Part model, mm, in its own coordinate system. Face numbers are marked on the shaded views. A direction names the side the tool comes from. Coordinates: 2 decimals unless noted, no trailing zeros. Write each loop counter-clockwise with the first axis right and the second up, starting at its lowest first coordinate (ties: lowest second). Pieces come first, ordered by that corner, then holes. Notation, with made-up numbers: (8.25, 35.25) - (25.25, 35.25) arc R29 ccw to (25.25, 62.25) - close; hole circle Ø11 at (-15, 45.5). An arc over 180 degrees is marked (long way). Use a Markdown table: item, result.
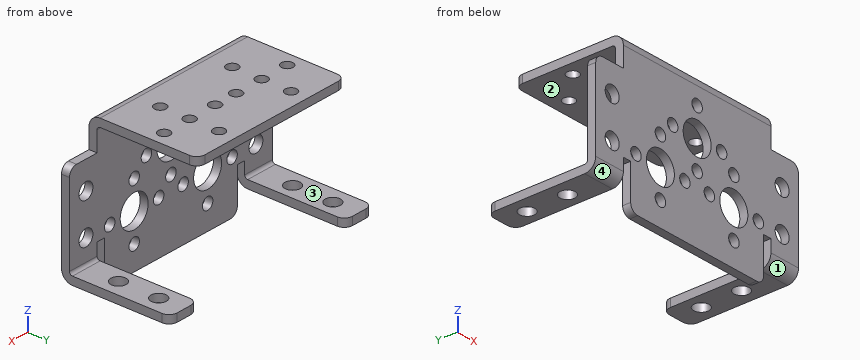
```python
from build123d import *

# Parameters (mm, degrees)
SM_BASE_FLANGE_1_DEPTH             = 2
SM_EDGE_FLANGE_1_STRIP_W           = 9.4732
SM_EDGE_FLANGE_1_STRIP_H           = 2
SM_EDGE_FLANGE_1_STRIP_CUT_DEPTH   = 42.2
SM_EDGE_FLANGE_1_DEPTH             = 42.2
SM_START                           = 2
SM_EDGE_FLANGE_1_FLAT_DEPTH        = 2
SM_EDGE_FLANGE_2_STRIP_W           = 9.4732
SM_EDGE_FLANGE_2_STRIP_H           = 2
SM_EDGE_FLANGE_2_STRIP_CUT_DEPTH   = 7.9
SM_EDGE_FLANGE_2_STRIP_2_W         = 9.4732
SM_EDGE_FLANGE_2_STRIP_2_H         = 2
SM_EDGE_FLANGE_2_STRIP_CUT_2_DEPTH = 7.9
SM_EDGE_FLANGE_2_DEPTH             = 7.9
SM_EDGE_FLANGE_2_PROFILE_R         = 1.9
SM_EDGE_FLANGE_2_FLAT_DEPTH        = 2
SM_EDGE_FLANGE_2_BEND_DEPTH        = 7.9
SM_EDGE_FLANGE_2_PROFILE_2_R       = 1.9
SM_EDGE_FLANGE_2_FLAT_2_DEPTH      = 2
HOLE_WIZARD_8_0_8_1_D              = 8
HOLE_WIZARD_3_0_3_1_D              = 3
HOLE_WIZARD_4_0_4_1_D              = 4
HOLE_WIZARD_2_9_2_9_2_D            = 2.9


# Sheet-metal steps are written as plain solids
with BuildPart() as part:
    # Sketch 2 → 基体-法兰1 (new body)
    with BuildSketch(Plane(origin=(0, 0, 0), x_dir=(1, 0, 0), z_dir=(0, 1, 0))):
        with BuildLine():
            Line((-17, 23.49), (17, 23.49))
            ThreePointArc((17, 23.49), (18.414213562, 22.904213562), (19, 21.49))
            Line((19, 21.49), (19, 12.7))
            Line((19, 12.7), (21.1, 12.7))
            Line((21.1, 12.7), (21.1, 16.5))
            Line((21.1, 16.5), (29, 16.5))
            Line((29, 16.5), (29, -4.3))
            ThreePointArc((29, -4.3), (28.414213562, -5.714213562), (27, -6.3))
            Line((27, -6.3), (21.1, -6.3))
            Line((21.1, -6.3), (21.1, -12))
            Line((21.1, -12), (-21.1, -12))
            Line((-21.1, -12), (-21.1, -6.3))
            Line((-21.1, -6.3), (-27, -6.3))
            ThreePointArc((-27, -6.3), (-28.414213562, -5.714213562), (-29, -4.3))
            Line((-29, -4.3), (-29, 16.5))
            Line((-29, 16.5), (-21.1, 16.5))
            Line((-21.1, 16.5), (-21.1, 12.7))
            Line((-21.1, 12.7), (-19, 12.7))
            Line((-19, 12.7), (-19, 21.49))
            ThreePointArc((-19, 21.49), (-18.414213562, 22.904213562), (-17, 23.49))
        make_face()
    extrude(amount=-SM_BASE_FLANGE_1_DEPTH)

    # 边线-法兰1 strip (across the edge) → 边线-法兰1 strip cut (cut)
    with BuildSketch(Plane(origin=(-21.1, 0, 12), x_dir=(0, 0, -1), z_dir=(1, 0, 0))):
        with Locations((-4, -1)):
            Rectangle(SM_EDGE_FLANGE_1_STRIP_W, SM_EDGE_FLANGE_1_STRIP_H)
    extrude(amount=SM_EDGE_FLANGE_1_STRIP_CUT_DEPTH, mode=Mode.SUBTRACT)

    # 边线-法兰1 bend section (across the edge) → 边线-法兰1 (add)
    with BuildSketch(Plane(origin=(-21.1, 0, 12), x_dir=(0, 0, -1), z_dir=(1, 0, 0))):
        with BuildLine():
            Line((-2, 0.7366), (0, 0.7366))
            ThreePointArc((0, 0.7366), (0.215745145, 0.215745145), (0.7366, 0))
            Line((0.7366, 0), (0.7366, -2))
            ThreePointArc((0.7366, -2), (-1.198468417, -1.198468417), (-2, 0.7366))
        make_face()
    extrude(amount=SM_EDGE_FLANGE_1_DEPTH)

    # 边线-法兰1 profile (on flange) → 边线-法兰1 flat (add)
    with BuildSketch(Plane.XY.offset(12).offset(SM_START)):
        with BuildLine():
            Line((-21.1, 0.7366), (21.1, 0.7366))
            Line((21.1, 0.7366), (21.1, 23))
            ThreePointArc((21.1, 23), (20.514213562, 24.414213562), (19.1, 25))
            Line((19.1, 25), (-19.1, 25))
            ThreePointArc((-19.1, 25), (-20.514213562, 24.414213562), (-21.1, 23))
            Line((-21.1, 23), (-21.1, 0.7366))
        make_face()
    extrude(amount=-SM_EDGE_FLANGE_1_FLAT_DEPTH)

    # 边线-法兰2 strip (across the edge) → 边线-法兰2 strip cut (cut)
    with BuildSketch(Plane(origin=(-21.1, 0, -16.5), x_dir=(0, 0, 1), z_dir=(-1, 0, 0))):
        with Locations((-4, -1)):
            Rectangle(SM_EDGE_FLANGE_2_STRIP_W, SM_EDGE_FLANGE_2_STRIP_H)
    extrude(amount=SM_EDGE_FLANGE_2_STRIP_CUT_DEPTH, mode=Mode.SUBTRACT)

    # 边线-法兰2 strip 2 (across the edge) → 边线-法兰2 strip cut 2 (cut)
    with BuildSketch(Plane(origin=(29, 0, -16.5), x_dir=(0, 0, 1), z_dir=(-1, 0, 0))):
        with Locations((-4, -1)):
            Rectangle(SM_EDGE_FLANGE_2_STRIP_2_W, SM_EDGE_FLANGE_2_STRIP_2_H)
    extrude(amount=SM_EDGE_FLANGE_2_STRIP_CUT_2_DEPTH, mode=Mode.SUBTRACT)

    # 边线-法兰2 bend section (across the edge) → 边线-法兰2 (add)
    with BuildSketch(Plane(origin=(-21.1, 0, -16.5), x_dir=(0, 0, 1), z_dir=(-1, 0, 0))):
        with BuildLine():
            Line((-2, 0.7366), (0, 0.7366))
            ThreePointArc((0, 0.7366), (0.215745145, 0.215745145), (0.7366, 0))
            Line((0.7366, 0), (0.7366, -2))
            ThreePointArc((0.7366, -2), (-1.198468417, -1.198468417), (-2, 0.7366))
        make_face()
    extrude(amount=SM_EDGE_FLANGE_2_DEPTH)

    # 边线-法兰2 profile (on flange) → 边线-法兰2 flat (add)
    with BuildSketch(Plane(origin=(0, 0, -16.5), x_dir=(-1, 0, 0), z_dir=(0, 0, -1)).offset(SM_START)):
        with BuildLine():
            ThreePointArc((23.1, 25), (21.685786438, 24.414213562), (21.1, 23))
            Line((21.1, 23), (21.1, 0.7366))
            Line((21.1, 0.7366), (29, 0.7366))
            Line((29, 0.7366), (29, 23))
            ThreePointArc((29, 23), (28.414213562, 24.414213562), (27, 25))
            Line((27, 25), (23.1, 25))
        make_face()
        with Locations((24.9, 8.6)):
            Circle(SM_EDGE_FLANGE_2_PROFILE_R, mode=Mode.SUBTRACT)
        with Locations((24.9, 18.6)):
            Circle(SM_EDGE_FLANGE_2_PROFILE_R, mode=Mode.SUBTRACT)
    extrude(amount=-SM_EDGE_FLANGE_2_FLAT_DEPTH)

    # 边线-法兰2 bend section 2 (across the edge) → 边线-法兰2 bend (add)
    with BuildSketch(Plane(origin=(29, 0, -16.5), x_dir=(0, 0, 1), z_dir=(-1, 0, 0))):
        with BuildLine():
            Line((-2, 0.7366), (0, 0.7366))
            ThreePointArc((0, 0.7366), (0.215745145, 0.215745145), (0.7366, 0))
            Line((0.7366, 0), (0.7366, -2))
            ThreePointArc((0.7366, -2), (-1.198468417, -1.198468417), (-2, 0.7366))
        make_face()
    extrude(amount=SM_EDGE_FLANGE_2_BEND_DEPTH)

    # 边线-法兰2 profile 2 (on flange) → 边线-法兰2 flat 2 (add)
    with BuildSketch(Plane(origin=(0, 0, -16.5), x_dir=(-1, 0, 0), z_dir=(0, 0, -1)).offset(SM_START)):
        with BuildLine():
            Line((-29, 23), (-29, 0.7366))
            Line((-29, 0.7366), (-21.1, 0.7366))
            Line((-21.1, 0.7366), (-21.1, 23))
            ThreePointArc((-21.1, 23), (-21.685786438, 24.414213562), (-23.1, 25))
            Line((-23.1, 25), (-27, 25))
            ThreePointArc((-27, 25), (-28.414213562, 24.414213562), (-29, 23))
        make_face()
        with Locations((-24.9, 8.6)):
            Circle(SM_EDGE_FLANGE_2_PROFILE_2_R, mode=Mode.SUBTRACT)
        with Locations((-24.9, 18.6)):
            Circle(SM_EDGE_FLANGE_2_PROFILE_2_R, mode=Mode.SUBTRACT)
    extrude(amount=-SM_EDGE_FLANGE_2_FLAT_2_DEPTH)

    # Ø8.0 (8) 直径孔1 (through all)
    with Locations(Plane(origin=(0, 0, 0), x_dir=(1, 0, 0), z_dir=(0, 1, 0))):
        with Locations((0, 0), (-10.5, 10.5), (10.5, 10.5)):
            Hole(HOLE_WIZARD_8_0_8_1_D / 2)

    # Ø3.0 (3) 直径孔1 (through all)
    with Locations(Plane(origin=(0, 0, 0), x_dir=(1, 0, 0), z_dir=(0, 1, 0))):
        with Locations((0, -7), (-17.5, 10.5), (17.5, 10.5), (-3.5, 10.5), (-10.5, 17.5), (-10.5, 3.5), (0, 7), (-7, 0), (7, 0), (10.5, 3.5), (3.5, 10.5), (10.5, 17.5)):
            Hole(HOLE_WIZARD_3_0_3_1_D / 2)

    # Ø4.0 (4) 直径孔1 (through all)
    with Locations(Plane(origin=(0, 0, 0), x_dir=(1, 0, 0), z_dir=(0, 1, 0))):
        with Locations((-24.3, 10.5), (-24.3, 0.5), (24.3, 10.5), (24.3, 0.5)):
            Hole(HOLE_WIZARD_4_0_4_1_D / 2)

    # Ø2.9 (2.9) 直径孔2 (through all)
    with Locations(Plane.XY.offset(14)):
        with Locations((10.3, 13.6), (-10.3, 13.6), (-10.3, 20.9), (-17.6, 13.6), (-10.3, 6.3), (-3, 13.6), (3, 13.6), (10.3, 20.9), (10.3, 6.3), (17.6, 13.6)):
            Hole(HOLE_WIZARD_2_9_2_9_2_D / 2)


solid = part.part
```
Item 1: Band-saw the part on B-B, the plane x = -17.6. Give the cut face in (y, z), then the cut area to 3 significant figures.
From the geometry:
| item | result |
|---|---|
| outline | (-2, -23.4) - (0, -23.4) - (0, -12) - (-2, -12) - close; (-2, -9) - (0, -9) - (0, 11.26) arc R0.74 cw to (0.74, 12) - (12.15, 12) - (12.15, 14) - (0.74, 14) arc R2.74 ccw to (-2, 11.26) - close; (15.05, 12) - (25, 12) - (25, 14) - (15.05, 14) - close |
| area | 112 mm^2 |
Item 2: Band-saw the part on D-D, the plane x = -3. Give the cut face in (y, z), then the cut area to 3 significant figures.
From the geometry:
| item | result |
|---|---|
| outline | (-2, -23.49) - (0, -23.49) - (0, -11.91) - (-2, -11.91) - close; (-2, -9.09) - (0, -9.09) - (0, -2.65) - (-2, -2.65) - close; (-2, 2.65) - (0, 2.65) - (0, 11.26) arc R0.74 cw to (0.74, 12) - (12.15, 12) - (12.15, 14) - (0.74, 14) arc R2.74 ccw to (-2, 11.26) - close; (15.05, 12) - (25, 12) - (25, 14) - (15.05, 14) - close |
| area | 101 mm^2 |
Item 3: Drill centre lines: probe 1 along X at (y, z) = (-0.75, -17.5); probe 2 along Y at (x, z) = (1, -22); probe 3 along Z at (x, y) = (-10.5, -1.1). Where is each one in solid material? Low to high.
From the geometry:
| item | result |
|---|---|
| probe 1 | -29 to -21.1, -19 to -12, -9 to 9, 12 to 19, 21.1 to 29 |
| probe 2 | -2 to 0 |
| probe 3 | -23.49 to -19, -16 to -14.5, -6.5 to -5, -2 to 13.29 |
Item 4: Drop flat-ended pins along their axis: P1, Ø1, axis at x = -20, y = -1.5, coming from the -Z side; P2, Ø12, axis at x = -4, y = 13.5, coming from the -Z side; P3, Ø5, axis at x = 10.5, z = -3.5, coming from the +Y side; P4, Ø3.5, axis at x = -24.9, y = 18.6, coming from the -Z side. Give the stop position or say it passes through.
From the geometry:
| item | result |
|---|---|
| P1 | z = -12.7 |
| P2 | z = 12 |
| P3 | y = 0 |
| P4 | through |
Item 5: Which spindle directions (+Z, -Z, +X, -X, +Y, -Y) get a long thin tool onto all of the face, cutting with end or side? Do the marked faces 1, 2, 3 and 4. Say none if no direction does.
From the geometry:
| item | result |
|---|---|
| face 1 | -Z, +X, -Y |
| face 2 | -Z, +X, -X, +Y |
| face 3 | +Z, +X, -X, +Y |
| face 4 | -Z, -X, -Y |
Item 6: Band-saw the part on C-C, the plane y = 17.75. Give the cut face in (x, z).
From the geometry:
| item | result |
|---|---|
| outline | (-29, -18.5) - (-26.6, -18.5) - (-26.6, -16.5) - (-29, -16.5) - close; (-23.2, -18.5) - (-21.1, -18.5) - (-21.1, -16.5) - (-23.2, -16.5) - close; (-21.1, 12) - (21.1, 12) - (21.1, 14) - (-21.1, 14) - close; (21.1, -18.5) - (23.2, -18.5) - (23.2, -16.5) - (21.1, -16.5) - close; (26.6, -18.5) - (29, -18.5) - (29, -16.5) - (26.6, -16.5) - close |
Item 7: Band-saw the part on A-A, the plane z = 7. Give the cut face in (x, y).
From the geometry:
| item | result |
|---|---|
| outline | (-21.1, -2) - (-1.5, -2) - (-1.5, 0) - (-21.1, 0) - close; (1.5, -2) - (21.1, -2) - (21.1, 0) - (1.5, 0) - close |
